Autodesk Inventor part; units mm, degrees
ref_plane "YZ Plane" through (0, 0, 0) normal (1, 0, 0) x (0, 1, 0)
ref_plane "XZ Plane" through (0, 0, 0) normal (0, 1, 0) x (-1, 0, 0)
ref_plane "XY Plane" through (0, 0, 0) normal (0, 0, 1) x (1, 0, 0)
sketch "Sketch1" plane through (0, 0, 0) normal (0, 0, 1) x (1, 0, 0)
  line L0 (-29.8485, 74.7727) -> (10.1515, 74.7727)
  line L1 (10.1515, 74.7727) -> (10.1515, -55.2273)
  line L2 (10.1515, -55.2273) -> (-29.8485, -55.2273)
  line L3 (-29.8485, -55.2273) -> (-29.8485, 74.7727)
  point P0 (0, 0)
  dimension "d0" = 40
  dimension "d1" = 130
extrude "Extrusion1" add sketch "Sketch1" along normal blind 6
sketch "Sketch2" plane through (0, 0, 0) normal (0, 0, -1) x (-1, 0, 0)
  circle A0 centre (9.8485, 58.7727) radius 3.3
  circle A1 centre (9.8485, 4.7727) radius 3.3
  point P0 (0, 0)
extrude "Extrusion2" cut sketch "Sketch2" against normal through all
sketch "Sketch3" plane through (0, 0, 0) normal (0, 0, -1) x (-1, 0, 0)
  line L0 (-10.1515, 74.7727) -> (-10.1515, -55.2273)
  line L1 (29.8485, -55.2273) -> (29.8485, 74.7727)
  line L2 (-10.1515, 74.7727) -> (29.8485, 74.7727)
  line L3 (29.8485, 74.7727) -> (29.8485, 68.7727)
  line L4 (29.8485, 68.7727) -> (-10.1515, 68.7727)
  line L5 (-10.1515, 68.7727) -> (-10.1515, 74.7727)
  line L6 (-10.1515, -55.2273) -> (-10.1515, 74.7727)
  line L7 (29.8485, -55.2273) -> (-10.1515, -55.2273)
  line L8 (-10.1515, -55.2273) -> (-10.1515, -49.2273)
  line L9 (-10.1515, -49.2273) -> (29.8485, -49.2273)
  line L10 (29.8485, -49.2273) -> (29.8485, -55.2273)
  point P0 (0, 0)
  dimension "d6" = 6
  dimension "d7" = 6
extrude "Extrusion3" add sketch "Sketch3" along normal blind 3 contours L2 L1 L4 L0 | L9 L1 L7 L0
sketch "Sketch4" plane through (0, 0, -3) normal (0, 0, -1) x (-1, 0, 0)
  line L0 (-10.1515, 68.7727) -> (29.8485, 68.7727)
  line L1 (-10.1515, 68.7727) -> (29.8485, 68.7727)
  line L2 (29.8485, 68.7727) -> (29.8485, 102.7727)
  line L3 (29.8485, 102.7727) -> (-10.1515, 102.7727)
  line L4 (-10.1515, 102.7727) -> (-10.1515, 68.7727)
  line L5 (29.8485, -49.2273) -> (-10.1515, -49.2273)
  line L6 (29.8485, -49.2273) -> (-10.1515, -49.2273)
  line L7 (-10.1515, -49.2273) -> (-10.1515, -114.2273)
  line L8 (-10.1515, -114.2273) -> (29.8485, -114.2273)
  line L9 (29.8485, -114.2273) -> (29.8485, -49.2273)
  point P0 (0, 0)
  dimension "d10" = 34
  dimension "d11" = 65
  dimension "d12" = 40
  dimension "d13" = 40
extrude "Extrusion4" add sketch "Sketch4" along normal blind 6
fillet "Fillet1" radius 3 8 edges at (-9.8485, 68.7727, 0) (-9.8485, 68.7727, -9) (-9.8485, 74.7727, -3) (-9.8485, 74.7727, 6) (-9.8485, -49.2273, 0) (-9.8485, -49.2273, -9) (-9.8485, -55.2273, -3) (-9.8485, -55.2273, 6)
sketch "Sketch5" plane through (0, 0, -9) normal (0, 0, -1) x (-1, 0, 0)
  circle A0 centre (11.3485, 91.2727) radius 4
  circle A1 centre (-2.6515, 91.2727) radius 4
  circle A2 centre (-2.6515, 91.2727) radius 4
  circle A3 centre (11.3485, 91.2727) radius 4
  circle A4 centre (-2.6515, 91.2727) radius 4
  circle A5 centre (11.3485, 91.2727) radius 4
  circle A6 centre (7.3485, -80.7273) radius 4
  circle A7 centre (7.3483, -96.165) radius 4
  point P0 (0, 0)
extrude "Extrusion5" cut sketch "Sketch5" against normal through all
properties part number "Ball screw right hand support"
Build history of the part. All positions in model axes, mm. A direction names the side the tool comes from. Give positions to 0.01 mm unless a question says otherwise; leave off trailing zeros. Write each loop counter-clockwise with the first axis right and the second up, starting at its lowest first coordinate (ties: lowest second). Pieces come first, ordered by that corner, then holes. Notation, with made-up numbers: (74, 24.25) - (96, 24.25) arc R20 cw to (96, 34.25) - close; hole circle Ø11 at (70, 55.5). An arc over 180 degrees is marked (long way). Use one line per item in the form item = value. Start each with the question number.
1. Two-plate mould, pull along X, no slides. Class faces 6 (the face through (-10, 11, 6)), 7 (the face through (10.152, -4, 2)), 8 (the face through (-29.848, -7, 2)), 9 (the face through (-9.419, 8.045, 2.958)): released by +X, released by -X, zero draft, split by the parting line, or undercut.
2. Band-saw the part on A-A on x = -26.5. Write the cut outline in (y, z), plus the area to 3 significant figures.
3. Probe line 1 (Y direction, x = -18, z = -3.25); line 2 (Y direction, x = -9, z = 3.75); line 3 (Z direction, x = 5, y = -15). List the from-to ranges inside material, lowest first. Write a range as [from, to].
4. 3-axis set-ups, long thin cutter, end or side, ignore diameter. For faces 1 (the face through (-14, 88, -3)), 2 (the face through (-10, -114.227, -6)), 3 (the face through (-10, -86, -3)), 4 (the face through (-10, 87, -9)), 5 (the face through (-10, 11, 0)): which of +Z, -Z, +X, -X, +Y, -Y reach the whole face in a straight line?
5. Band-saw the part on B-B on y = -35. Write the cut outline in (x, z).
6. Drop flat-ended pins along their axis: pin 1 Ø6 at (x, y) = (-9.85, 4.77) entering from +Z; pin 2 Ø6 at (x, z) = (1, 2) entering from -Y; pin 3 Ø2.5 at (x, z) = (-3, 1.5) entering from -Y; pin 4 Ø4 at (x, z) = (-12.5, 0) entering from -Y. Give the stop position or say it passes through.
Conclusion:
q1.face_6 = zero draft
q1.face_7 = released by +X
q1.face_8 = released by -X
q1.face_9 = undercut
q2.outline = (-114.23, -9) - (-52.23, -9) arc R3 ccw to (-49.23, -6) - (-49.23, -3) arc R3 cw to (-46.23, 0) - (65.77, 0) arc R3 cw to (68.77, -3) - (68.77, -6) arc R3 ccw to (71.77, -9) - (102.77, -9) - (102.77, -3) - (77.77, -3) arc R3 cw to (74.77, 0) - (74.77, 3) arc R3 ccw to (71.77, 6) - (-52.23, 6) arc R3 ccw to (-55.23, 3) - (-55.23, 0) arc R3 cw to (-58.23, -3) - (-114.23, -3) - close
q2.area = 1,410 mm²
q3.line_1 = [-114.23, -49.23], [68.77, 102.77]
q3.line_2 = [-55.13, 1.58], [7.96, 55.58], [61.96, 74.68]
q3.line_3 = [0, 6]
q4.face_1 = +Z, +X, -X, +Y
q4.face_2 = +Z, -Z, +X, -X, -Y
q4.face_3 = +Z, +X, -X, -Y
q4.face_4 = -Z, +X, -X, +Y, -Y
q4.face_5 = -Z, +X, -X
q5.outline = (-29.85, 0) - (10.15, 0) - (10.15, 6) - (-29.85, 6) - close
q6.pin_1 = through
q6.pin_2 = -55.4
q6.pin_3 = -55.23
q6.pin_4 = -55.99
